```python
from build123d import *

# Parameters (mm, degrees)
SKETCH_W  = 100
SKETCH_H  = 100
PAD_DEPTH = 10


with BuildPart() as part:
    # Sketch → Pad (new body)
    with BuildSketch(Plane.XY):
        Rectangle(SKETCH_W, SKETCH_H)
    extrude(amount=PAD_DEPTH)

    # Cone → Cone (revolve)
    with BuildSketch(Plane(origin=(0, 0, 10), x_dir=(1, 0, 0), z_dir=(0, -1, 0))):
        Polygon((0, 0), (25, 0), (10, 50), (0, 50), align=None)
    revolve(axis=Axis((0, 0, 10), (0, 0, 1)))


solid = part.part
```
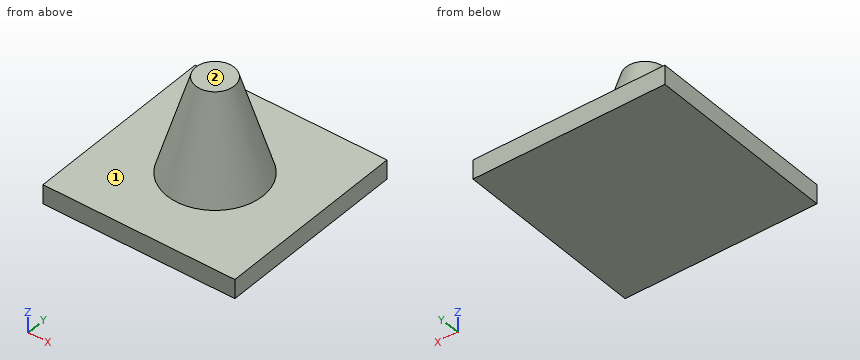
Source: CAD feature listing. Evaluate the final solid. Frame: model axes, mm. Face numbers are marked on the shaded views. A direction names the side the tool comes from. Coordinates: 2 decimals unless noted, no trailing zeros. Loops run counter-clockwise (first coordinate to the right, second up) from the corner with the lowest first, then second, coordinate; pieces in that order, holes last. Notation, with made-up numbers: (-2.75, 85.25) -> (25.25, 85.25) arc R30 ccw to (25.25, 114.25) -> close; hole circle Ø7 at (-1, 49). An arc over 180 degrees is marked (long way). One line per item, written item: value. Start each with the question number.
Q1. Set-up query: the marked faces 1 and 2. Return all of +Z, -Z, +X, -X, +Y, -Y with unobstructed straight access to the full face (end or side cutting, diameter ignored); none if empty.
Q2. Line query: line 1 along Z through (x, y) = (-10, -45); line 2 along Y through (x, z) = (-4.5, 31); line 3 along Y through (x, z) = (20, 18). Output: solid intervals per line, ascending.
Q3. Section query C-C, the plane z = 28.5. Return the cut outline in (x, y).
Q4. Section query A-A, the plane x = 0. Return the cut outline in (y, z), and give its area (3 significant figures).
Q5. Section query D-D, the plane z = 47. Return the cut outline in (x, y), and give its area (3 significant figures).
Q6. Contact query for flat-ended pins moving along their axis: P1, Ø4, axis at x = 2, z = 26.5, coming from the -Y side; P2, Ø2, axis at x = 15, y = 30.5, coming from the +Z side; P3, Ø8, axis at x = -6.5, z = 54, coming from the -Y side; P4, Ø12, axis at x = 28, z = 35.5, coming from the -Y side. Output: stop coordinate, or through.
Results:
1. face 1: +Z
1. face 2: +Z, +X, -X, +Y, -Y
2. line 1: 0 to 10
2. line 2: -18.15 to 18.15
2. line 3: -10.52 to 10.52
3. outline: circle Ø38.9 at (0, 0)
4. outline: (-50, 0) -> (50, 0) -> (50, 10) -> (25, 10) -> (10, 60) -> (-10, 60) -> (-25, 10) -> (-50, 10) -> close
4. area: 2,750 mm^2
5. outline: circle Ø27.8 at (0, 0)
5. area: 607 mm^2
6. P1: y = -20.58
6. P2: z = 10
6. P3: y = -12.1
6. P4: through
